from build123d import *

# Parameters (mm, degrees)
SKETCH1_W           = 121
SKETCH1_H           = 66
BOSS_EXTRUDE1_DEPTH = 3
SKETCH2_W           = 109
SKETCH2_H           = 58
CUT_EXTRUDE1_DEPTH  = 4
FILLET1_R           = 5
SKETCH3_W           = 20
SKETCH3_H           = 58
BOSS_EXTRUDE2_DEPTH = 3
FILLET2_R           = 3
SKETCH4_R           = 1
CUT_EXTRUDE2_DEPTH  = 4
BOSS_EXTRUDE3_DEPTH = 3
FILLET3_R           = 3
SKETCH6_W           = 3
SKETCH6_H           = 10
SKETCH6_W_2         = 10
SKETCH6_H_2         = 3
CUT_EXTRUDE3_DEPTH  = 4


with BuildPart() as part:
    # Sketch1 → Boss-Extrude1 (new body)
    with BuildSketch(Plane(origin=(0, 0, 0), x_dir=(1, 0, 0), z_dir=(0, 1, 0))):
        with Locations((60.5, -33)):
            Rectangle(SKETCH1_W, SKETCH1_H)
    extrude(amount=BOSS_EXTRUDE1_DEPTH)

    # Sketch2 → Cut-Extrude1 (cut, through all)
    with BuildSketch(Plane(origin=(0, 3, 0), x_dir=(1, 0, 0), z_dir=(0, 1, 0))):
        with Locations((60.5, -33)):
            Rectangle(SKETCH2_W, SKETCH2_H)
    extrude(amount=-CUT_EXTRUDE1_DEPTH, mode=Mode.SUBTRACT)

    # Fillet1
    fillet1_edges = [part.edges().sort_by_distance(p)[0] for p in [
        (115, 1.5, 4),
        (115, 1.5, 62),
        (6, 1.5, 62),
        (6, 1.5, 4),
    ]]
    fillet(fillet1_edges, radius=FILLET1_R)

    # Sketch3 → Boss-Extrude2 (add, through all)
    with BuildSketch(Plane(origin=(0, 3, 0), x_dir=(1, 0, 0), z_dir=(0, 1, 0))):
        with Locations((60.5, -33)):
            Rectangle(SKETCH3_W, SKETCH3_H)
    extrude(amount=-BOSS_EXTRUDE2_DEPTH)

    # Fillet2
    fillet2_edges = [part.edges().sort_by_distance(p)[0] for p in [
        (70.5, 1.5, 4),
        (70.5, 1.5, 62),
        (50.5, 1.5, 62),
        (50.5, 1.5, 4),
    ]]
    fillet(fillet2_edges, radius=FILLET2_R)

    # Sketch4 → Cut-Extrude2 (cut, through all)
    with BuildSketch(Plane(origin=(0, 3, 0), x_dir=(1, 0, 0), z_dir=(0, 1, 0))):
        with Locations((116.5, -61.5)):
            Circle(SKETCH4_R)
        with Locations((116.5, -4.5)):
            Circle(SKETCH4_R)
        with Locations((4.5, -4.5)):
            Circle(SKETCH4_R)
        with Locations((4.5, -61.5)):
            Circle(SKETCH4_R)
    extrude(amount=-CUT_EXTRUDE2_DEPTH, mode=Mode.SUBTRACT)

    # Sketch5 → Boss-Extrude3 (add, through all)
    with BuildSketch(Plane(origin=(0, 3, 0), x_dir=(1, 0, 0), z_dir=(0, 1, 0))):
        Polygon((0, 0), (-15, 0), (-15, -76), (136, -76), (136, 0), (121, 0), (121, -66), (0, -66), align=None)
    extrude(amount=-BOSS_EXTRUDE3_DEPTH)

    # Fillet3
    fillet3_edges = [part.edges().sort_by_distance(p)[0] for p in [
        (136, 1.5, 0),
        (136, 1.5, 76),
        (-15, 1.5, 76),
        (-15, 1.5, 0),
    ]]
    fillet(fillet3_edges, radius=FILLET3_R)

    # Sketch6 → Cut-Extrude3 (cut, through all)
    with BuildSketch(Plane.XZ):
        with Locations((131.5, 25)):
            Rectangle(SKETCH6_W, SKETCH6_H)
        with Locations((131.5, 45)):
            Rectangle(SKETCH6_W, SKETCH6_H)
        with Locations((131.5, 65)):
            Rectangle(SKETCH6_W, SKETCH6_H)
        with Locations((120.5, 71.5)):
            Rectangle(SKETCH6_W_2, SKETCH6_H_2)
        with Locations((100.5, 71.5)):
            Rectangle(SKETCH6_W_2, SKETCH6_H_2)
        with Locations((80.5, 71.5)):
            Rectangle(SKETCH6_W_2, SKETCH6_H_2)
        with Locations((60.5, 71.5)):
            Rectangle(SKETCH6_W_2, SKETCH6_H_2)
        with Locations((40.5, 71.5)):
            Rectangle(SKETCH6_W_2, SKETCH6_H_2)
        with Locations((20.5, 71.5)):
            Rectangle(SKETCH6_W_2, SKETCH6_H_2)
        with Locations((0.5, 71.5)):
            Rectangle(SKETCH6_W_2, SKETCH6_H_2)
        with Locations((-10.5, 65)):
            Rectangle(SKETCH6_W, SKETCH6_H)
        with Locations((-10.5, 45)):
            Rectangle(SKETCH6_W, SKETCH6_H)
        with Locations((-10.5, 25)):
            Rectangle(SKETCH6_W, SKETCH6_H)
    extrude(amount=-CUT_EXTRUDE3_DEPTH, mode=Mode.SUBTRACT)


solid = part.part
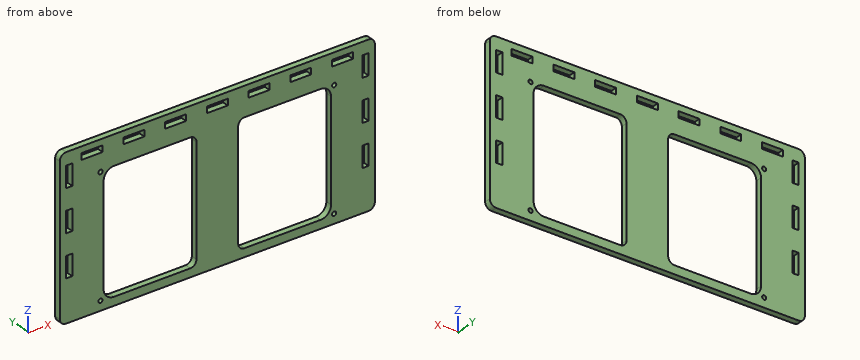
Geometry: final body of the model. Coordinates: model frame, mm. Round coordinates to 2 decimals unless told otherwise and drop trailing zeros. Loops run counter-clockwise (first coordinate to the right, second up) from the corner with the lowest first, then second, coordinate; pieces in that order, holes last. Notation, with made-up numbers: M 87,72.5 L 107,72.5 A19 ccw 107,89.5 Z; hole C 85.5,-33 d2. An arc over 180 degrees is marked long. One line per question, with ' | ' between items.
(1) Cut plane C-C on z = 12.5. Return the cut outline in (x, y).
Check result:
outline: M -15,0 L 6,0 L 6,3 L -15,3 Z; M 50.5,0 L 70.5,0 L 70.5,3 L 50.5,3 Z; M 115,0 L 136,0 L 136,3 L 115,3 Z
(2) Cut plane D-D on x = 33.5. Return the cut outline in (y, z).
Check result:
outline: M 0,0 L 3,0 L 3,4 L 0,4 Z; M 0,62 L 3,62 L 3,76 L 0,76 Z
(3) Material intervals for line 1 along Z through (x, y) = (4.5, 1.4); line 2 along Z through (x, y) = (84.5, 1.65); line 3 along X through (y, z) = (1.7, 29), sorted ascending. Write a range as from..to.
Check result:
line 1: z = 0..3.5, 5.5..60.5, 62.5..70, 73..76 | line 2: z = 0..4, 62..70, 73..76 | line 3: x = -15..-12, -9..6, 50.5..70.5, 115..130, 133..136
(4) Cut plane B-B on x = 59. Return the cut outline in (y, z), plus the area to 3 significant figures.
Check result:
outline: M 0,0 L 3,0 L 3,70 L 0,70 Z; M 0,73 L 3,73 L 3,76 L 0,76 Z | area: 219 mm2
(5) Contact query for a flat-ended pin moving along its axis: P1, Ø4, axis at x = 4, z = 38.5, coming from the -Y side. Output: stop coordinate, or through.
Check result:
P1: stops at y = 0
(6) Cut plane A-A on z = 23.5. Return the cut outline in (x, y).
Check result:
outline: M -15,0 L -12,0 L -12,3 L -15,3 Z; M -9,0 L 6,0 L 6,3 L -9,3 Z; M 50.5,0 L 70.5,0 L 70.5,3 L 50.5,3 Z; M 115,0 L 130,0 L 130,3 L 115,3 Z; M 133,0 L 136,0 L 136,3 L 133,3 Z
